Geometry check sheet. Reference: the model listing, model coordinates, mm. Face numbers are marked on the shaded views. A direction names the side the tool comes from. Give positions to 0.01 mm unless a question says otherwise; leave off trailing zeros. Loops run counter-clockwise (first coordinate to the right, second up) from the corner with the lowest first, then second, coordinate; pieces in that order, holes last. Notation, with made-up numbers: (74.5, 28.25) - (107.5, 28.25) arc R20 ccw to (107.5, 52.25) - close; hole circle Ø10 at (67.5, -30.75). An arc over 180 degrees is marked (long way). Use a Markdown table: item, result. Add a question column.
1. Cross-section at C-C on x = 0. Count the separate pieces of the cut face and the enclosed holes in it, and give its area (3 significant figures).
2. Cross-section at B-B on y = -5. Enter the section's corners in (x, z), and give its area (3 significant figures).
3. Depth check by flat-ended pin: P1, Ø3.5, axis at x = -0.5, z = 0.5, coming from the -Y side; P2, Ø1.5, axis at x = 4.5, z = 7.5, coming from the -Y side; P3, Ø6, axis at y = -7.5, z = 0, coming from the -X side. Enter the tip coordinate at first touch or a pass-through.
4. Material ranges on L1, parallel to Z at x = 0, y = -2; L2, parallel to Z at x = 0, y = 1.4; L3, parallel to Y at x = -3.5, z = 2.5, recorded low to high.
5. Draft check along Z on the marked faces 1, 2 and 3. Enter one of: pulls with the +Z half, pulls with the -Z half, needs draft (parallel to the pull), parting line crosses it, or undercut.
6. Cross-section at A-A on z = 10. Enter the section's corners in (x, y).
7. Set-up check for the marked faces 4, 5 and 6: record each of +Z, -Z, +X, -X, +Y, -Y from which the full face is reachable in a straight line by a thin tool's end or side.
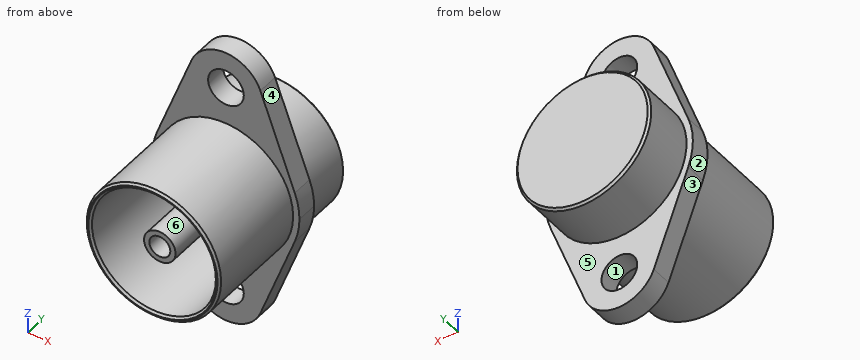
from build123d import *

# Parameters (mm, degrees)
F0_R     = 1.7
F0_R_2   = 6.4
F0_R_3   = 5.9
F0_R_4   = 1.5
F0_R_5   = 1
F1_DEPTH = 2
F2_DEPTH = 7
F3_DEPTH = 10
F4_DEPTH = 9
F6_SIZE  = 0.2


# Not quite as in the source:
# - the program builds the solid bodies; features that only make, move or delete a surface that nothing else refers to are left out


with BuildPart() as f1:
    # F0 (on Front) → F1 (new body)
    with BuildSketch(Plane.XZ):
        with BuildLine():
            Line((6.5572478983, 2.45), (3.2786239492, 11.225))
            ThreePointArc((3.2786239492, 11.225), (0, 13.5), (-3.2786239492, 11.225))
            Line((-3.2786239492, 11.225), (-6.5572478983, 2.45))
            ThreePointArc((-6.5572478983, 2.45), (0, 7), (6.5572478983, 2.45))
        make_face()
        with Locations((0, 10)):
            Circle(F0_R, mode=Mode.SUBTRACT)
        with BuildLine():
            ThreePointArc((6.5572478983, -2.45), (0, -7), (-6.5572478983, -2.45))
            Line((-6.5572478983, -2.45), (-3.2786239492, -11.225))
            ThreePointArc((-3.2786239492, -11.225), (0, -13.5), (3.2786239492, -11.225))
            Line((3.2786239492, -11.225), (6.5572478983, -2.45))
        make_face()
        with Locations((0, -10)):
            Circle(F0_R, mode=Mode.SUBTRACT)
        with BuildLine():
            ThreePointArc((7, 0), (6.8884227254, 1.2448423016), (6.5572478983, 2.45))
            ThreePointArc((6.5572478983, 2.45), (0, 7), (-6.5572478983, 2.45))
            ThreePointArc((-6.5572478983, 2.45), (-7, 0), (-6.5572478983, -2.45))
            ThreePointArc((-6.5572478983, -2.45), (0, -7), (6.5572478983, -2.45))
            ThreePointArc((6.5572478983, -2.45), (6.8884227254, -1.2448423016), (7, 0))
        make_face()
        Circle(F0_R_2, mode=Mode.SUBTRACT)
        Circle(F0_R_2)
        Circle(F0_R_3, mode=Mode.SUBTRACT)
        Circle(F0_R_3)
        Circle(F0_R_4, mode=Mode.SUBTRACT)
        Circle(F0_R_4)
        Circle(F0_R_5, mode=Mode.SUBTRACT)
        Circle(F0_R_5)
    extrude(amount=-F1_DEPTH)

    # F0 (on Front) → F2 (join)
    with BuildSketch(Plane.XZ):
        Circle(F0_R_2)
        Circle(F0_R_3, mode=Mode.SUBTRACT)
        Circle(F0_R_3)
        Circle(F0_R_4, mode=Mode.SUBTRACT)
        Circle(F0_R_4)
        Circle(F0_R_5, mode=Mode.SUBTRACT)
        Circle(F0_R_5)
    extrude(amount=-F2_DEPTH)

    # F0 (on Front) → F3 (join)
    with BuildSketch(Plane.XZ):
        Circle(F0_R_2)
        Circle(F0_R_3, mode=Mode.SUBTRACT)
    extrude(amount=F3_DEPTH)

    # F0 (on Front) → F4 (join)
    with BuildSketch(Plane.XZ):
        Circle(F0_R_4)
        Circle(F0_R_5, mode=Mode.SUBTRACT)
    extrude(amount=F4_DEPTH)

    # F6
    f6_edges = [f1.edges().sort_by_distance(p)[0] for p in [
        (-6.4, -10, 0),
        (-5.9, -10, 0),
        (-6.4, 7, 0),
    ]]
    chamfer(f6_edges, length=F6_SIZE)


solid = f1.part
Values found:
| question | item | result |
|---|---|---|
| 1 | separate pieces | 3 |
| 1 | enclosed holes | 0 |
| 1 | area | 123 mm2 |
| 2 | outline | circle Ø12.8 at (0, 0); circle Ø3 at (0, 0); hole circle Ø11.8 at (0, 0); hole circle Ø2 at (0, 0) |
| 2 | area | 23.2 mm2 |
| 3 | P1 | stops at y = -9 |
| 3 | P2 | stops at y = 0 |
| 3 | P3 | stops at x = -6.4 |
| 4 | L1 | z = -6.4 to -5.9, -1.5 to -1, 1 to 1.5, 5.9 to 6.4 |
| 4 | L2 | z = -13.5 to -11.7, -8.3 to 8.3, 11.7 to 13.5 |
| 4 | L3 | y = 0 to 7 |
| 5 | face 1 | undercut |
| 5 | face 2 | parting line crosses it |
| 5 | face 3 | pulls with the -Z half |
| 6 | outline | (-3.74, 0) - (-1.7, 0) - (-1.7, 2) - (-3.74, 2) - close; (1.7, 0) - (3.74, 0) - (3.74, 2) - (1.7, 2) - close |
| 7 | face 4 | +Z, +X, +Y, -Y |
| 7 | face 5 | +Y |
| 7 | face 6 | -Y |
